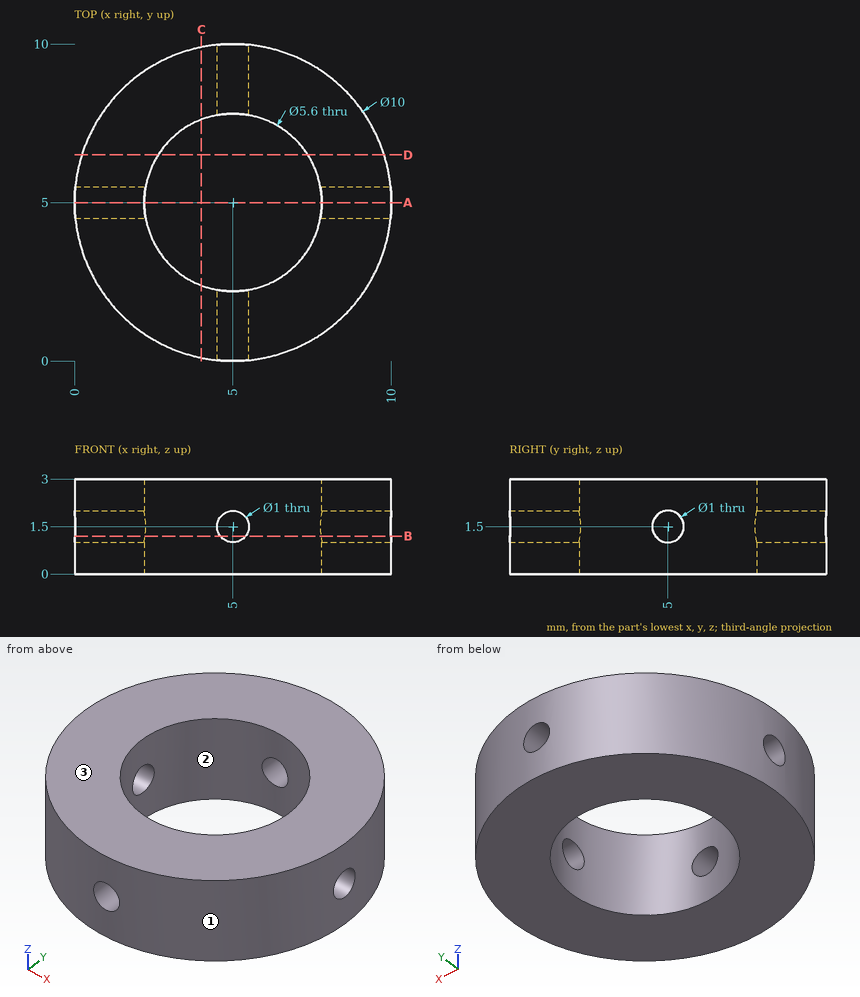
Geometry check sheet. Reference: drawing and pictorial views, mm from the part's lowest x, y, z. Round coordinates to 2 decimals unless told otherwise and drop trailing zeros. Loops run counter-clockwise (first coordinate to the right, second up) from the corner with the lowest first, then second, coordinate; pieces in that order, holes last. Notation, with made-up numbers: (63.25, 89.25) -> (67.25, 89.25) arc R24 ccw to (67.25, 117.25) -> close; hole circle Ø1 at (-31, 25). An arc over 180 degrees is marked (long way). Use a Markdown table: item, result.
(1) Sectioned sample at B-B (z = 1.2). Enter the section's corners in (x, y), then the cut area to 3 significant figures.
Calculated:
| item | result |
|---|---|
| outline | (0.02, 4.6) arc R5 ccw to (4.6, 0.02) -> (4.6, 2.23) arc R2.8 cw to (2.23, 4.6) -> close; (0.02, 5.4) -> (2.23, 5.4) arc R2.8 cw to (4.6, 7.77) -> (4.6, 9.98) arc R5 ccw to start; (5.4, 0.02) arc R5 ccw to (9.98, 4.6) -> (7.77, 4.6) arc R2.8 cw to (5.4, 2.23) -> close; (5.4, 7.77) arc R2.8 cw to (7.77, 5.4) -> (9.98, 5.4) arc R5 ccw to (5.4, 9.98) -> close |
| area | 46.9 mm² |
(2) Sectioned sample at A-A (y = 5). Enter the section's corners in (x, z), then the cut area to 3 significant figures.
Calculated:
| item | result |
|---|---|
| outline | (0, 0) -> (2.2, 0) -> (2.2, 1) -> (0, 1) -> close; (0, 2) -> (2.2, 2) -> (2.2, 3) -> (0, 3) -> close; (7.8, 0) -> (10, 0) -> (10, 1) -> (7.8, 1) -> close; (7.8, 2) -> (10, 2) -> (10, 3) -> (7.8, 3) -> close |
| area | 8.80 mm² |
(3) Sectioned sample at C-C (x = 4). Enter the section's corners in (y, z).
Calculated:
| item | result |
|---|---|
| outline | (0.1, 0) -> (2.38, 0) -> (2.38, 3) -> (0.1, 3) -> close; (7.62, 0) -> (9.9, 0) -> (9.9, 3) -> (7.62, 3) -> close |
(4) Mould release check, pull along Y, two halves, no side actions. Record for the marked faces 1, 2 and 3: released by +Y, released by -Y, zero draft, split by the parting line, or undercut.
Calculated:
| item | result |
|---|---|
| face 1 | split by the parting line |
| face 2 | undercut |
| face 3 | zero draft |
(5) Sectioned sample at D-D (y = 6.5). Enter the section's corners in (x, z), then the cut area to 3 significant figures.
Calculated:
| item | result |
|---|---|
| outline | (0.23, 0) -> (2.64, 0) -> (2.64, 3) -> (0.23, 3) -> close; (7.36, 0) -> (9.77, 0) -> (9.77, 3) -> (7.36, 3) -> close |
| area | 14.4 mm² |
(6) Scan lines: probe 1 along Z at (x, y) = (5, 0.5); probe 2 along Y at (x, z) = (5, 2.2); probe 3 along Y at (x, z) = (1.3, 1.5). Record each from-to range of solid material in increasing order.
Calculated:
| item | result |
|---|---|
| probe 1 | 0 to 1, 2 to 3 |
| probe 2 | 0 to 2.2, 7.8 to 10 |
| probe 3 | 1.64 to 4.5, 5.5 to 8.36 |
(7) Go/stop test with a flat-tipped pin: P1, Ø1, axis at x = 7.5, z = 0.5, coming from the -Y side. Record where the tip stops, or that it passes through.
Calculated:
| item | result |
|---|---|
| P1 | y = 0.42 |
